```python
from build123d import *

# Parameters (mm, degrees)
SKETCH1_W           = 100
SKETCH1_H           = 45
BOSS_EXTRUDE1_DEPTH = 19.5
SKETCH2_R           = 4
CUT_EXTRUDE1_DEPTH  = 46
SKETCH4_R           = 2.75
CUT_EXTRUDE3_DEPTH  = 20.5
SKETCH5_W           = 18
SKETCH5_H           = 6.5
CUT_EXTRUDE5_DEPTH  = 46
SKETCH6_W           = 18
SKETCH6_H           = 10
CUT_EXTRUDE6_DEPTH  = 4
BOSS_EXTRUDE2_DEPTH = 4


with BuildPart() as part:
    # Sketch1 → Boss-Extrude1 (new body)
    with BuildSketch(Plane.XY):
        Rectangle(SKETCH1_W, SKETCH1_H)
    extrude(amount=BOSS_EXTRUDE1_DEPTH)

    # Sketch2 → Cut-Extrude1 (cut, through all)
    with BuildSketch(Plane(origin=(0, 22.5, 0), x_dir=(1, 0, 0), z_dir=(0, 1, 0))):
        with Locations((-30, -9.75)):
            Circle(SKETCH2_R)
        with Locations((30, -9.75)):
            Circle(SKETCH2_R)
    extrude(amount=-CUT_EXTRUDE1_DEPTH, mode=Mode.SUBTRACT)

    # Sketch4 → Cut-Extrude3 (cut, through all)
    with BuildSketch(Plane(origin=(0, 0, 0), x_dir=(-1, 0, 0), z_dir=(0, 0, -1))):
        with Locations((-42.034787685, 14.2)):
            Circle(SKETCH4_R)
        with Locations((-42.034787685, -14.2)):
            Circle(SKETCH4_R)
        with Locations((42.034787685, -14.2)):
            Circle(SKETCH4_R)
        with Locations((42.034787685, 14.2)):
            Circle(SKETCH4_R)
    extrude(amount=-CUT_EXTRUDE3_DEPTH, mode=Mode.SUBTRACT)

    # Sketch5 → Cut-Extrude5 (cut, through all)
    with BuildSketch(Plane(origin=(0, 22.5, 0), x_dir=(1, 0, 0), z_dir=(0, 1, 0))):
        with Locations((0, -6.35)):
            Rectangle(SKETCH5_W, SKETCH5_H)
    extrude(amount=-CUT_EXTRUDE5_DEPTH, mode=Mode.SUBTRACT)

    # Sketch6 → Cut-Extrude6 (cut)
    with BuildSketch(Plane(origin=(0, 0, 0), x_dir=(-1, 0, 0), z_dir=(0, 0, -1))):
        Rectangle(SKETCH6_W, SKETCH6_H)
    extrude(amount=-CUT_EXTRUDE6_DEPTH, mode=Mode.SUBTRACT)

    # Sketch7 → Boss-Extrude2 (add)
    with BuildSketch(Plane.XY.offset(19.5)):
        with BuildLine():
            Line((4, 10), (4, -10))
            ThreePointArc((4, -10), (0, -14), (-4, -10))
            Line((-4, -10), (-4, 10))
            ThreePointArc((-4, 10), (0, 14), (4, 10))
        make_face()
    extrude(amount=BOSS_EXTRUDE2_DEPTH)


solid = part.part
```
Read the model definition and answer for the solid it produces. Units are mm, in the model's axes. A direction names the side the tool comes from. Give positions to 0.01 mm unless a question says otherwise; leave off trailing zeros. Order: outer loops, then holes, each group sorted by start corner. A loop starts at its lowest first (then second) coordinate and runs counter-clockwise, first axis right, second up.
(1) Find section A-A (z = 16). Give the vertices of the cut face in (x, y), plus the area to 3 significant figures.
(2) For faces 1 (the flat face through (0, -5, 2)), 2 (the cylindrical face through (0, -14, 21)), 3 (the flat face through (4, 0, 21)), 4 (the flat face through (-4, 0, 21)), 5 (the cylindrical face through (0, 14, 21)), determine the directions among +Z, -Z, +X, -X, +Y, -Y from which every point of the face is accessible in a straight line to the end or side of a thin tool.
(3) Straight lines are drawn through the part: L1, parallel to X at y = -14.5, z = 16.5; L2, parallel to Z at x = -4.5, y = 18; L3, parallel to X at y = -13, z = 12.75. For each, find the intervals that lie inside material, in ascending order.
(4) Find section D-D (z = 21.75). Give the vertices of the cut face in (x, y).
(5) Find section C-C (x = -30). Give the vertices of the cut face in (y, z), plus the area to 4 significant figures.
(6) Find section B-B (x = -8). Give the vertices of the cut face in (y, z).
(7) For a pull along Z with two mould halves and no side action, classify faces 6 (the flat face through (0, 0, 23.5)), 7 (the flat face through (9, 0, 6)), 8 (the flat face through (-1, -22.5, 10)) as released by +Z, released by -Z, zero draft, split by the parting line, or undercut.
(8) Given pin 1 (10 mm diameter, centred on x = 29, y = -16, fed in from -Z); pin 2 (2 mm diameter, centred on y = 2, z = 22, fed in from -X); pin 3 (5 mm diameter, centred on x = 30, z = 9.75, fed in from -Y); pin 4 (6 mm diameter, centred on x = 22.5, y = -2, fed in from +Z), each flat-ended and moving along its own axis, determine where each tip first touches the part or whether it passes through.
Result sheet:
1. outline: (-50, -22.5) - (50, -22.5) - (50, 22.5) - (-50, 22.5) - close; hole circle Ø5.5 at (-42.03, -14.2); hole circle Ø5.5 at (-42.03, 14.2); hole circle Ø5.5 at (42.03, -14.2); hole circle Ø5.5 at (42.03, 14.2)
1. area: 4,400 mm2
2. face 1: -Z
2. face 2: +Z, -Y
2. face 3: +Z, +X, +Y, -Y
2. face 4: +Z, -X, +Y, -Y
2. face 5: +Z, +Y
3. L1: x = -50 to -44.77, -39.3 to 39.3, 44.77 to 50
3. L2: z = 0 to 3.1, 9.6 to 19.5
3. L3: x = -50 to -44.51, -39.56 to -32.65, -27.35 to 27.35, 32.65 to 39.56, 44.51 to 50
4. outline: (-4, -10) arc R4 ccw to (4, -10) - (4, 10) arc R4 ccw to (-4, 10) - close
5. outline: (-22.5, 0) - (22.5, 0) - (22.5, 5.75) - (-22.5, 5.75) - close; (-22.5, 13.75) - (22.5, 13.75) - (22.5, 19.5) - (-22.5, 19.5) - close
5. area: 517.5 mm2
6. outline: (-22.5, 0) - (-5, 0) - (-5, 3.1) - (-22.5, 3.1) - close; (-22.5, 9.6) - (22.5, 9.6) - (22.5, 19.5) - (-22.5, 19.5) - close; (5, 0) - (22.5, 0) - (22.5, 3.1) - (5, 3.1) - close
7. face 6: released by +Z
7. face 7: undercut
7. face 8: zero draft
8. pin 1: stops at z = 0
8. pin 2: stops at x = -4
8. pin 3: passes through
8. pin 4: stops at z = 19.5
